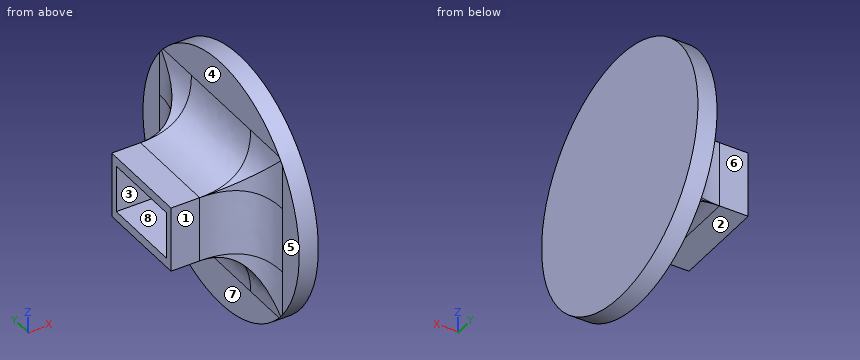
from build123d import *

# Parameters (mm, degrees)
SKETCH2_R           = 19.65
BOSS_EXTRUDE1_DEPTH = 3
SKETCH3_W           = 12.5
SKETCH3_H           = 14.9
BOSS_EXTRUDE2_DEPTH = 5.15
SKETCH4_W           = 7.4
SKETCH4_H           = 12.6
CUT_EXTRUDE1_DEPTH  = 12.5
FILLET1_SIZE        = 8


with BuildPart() as part:
    # Sketch2 → Boss-Extrude1 (new body)
    with BuildSketch(Plane(origin=(0, 0, 0), x_dir=(0, 0, -1), z_dir=(1, 0, 0))):
        Circle(SKETCH2_R)
    extrude(amount=BOSS_EXTRUDE1_DEPTH)

    # Sketch3 → Boss-Extrude2 (add, symmetric)
    with BuildSketch(Plane.XY):
        with Locations((-6.25, 0)):
            Rectangle(SKETCH3_W, SKETCH3_H)
    extrude(amount=BOSS_EXTRUDE2_DEPTH, both=True)

    # Sketch4 → Cut-Extrude1 (cut)
    with BuildSketch(Plane.ZY.offset(12.5)):
        Rectangle(SKETCH4_W, SKETCH4_H)
    extrude(amount=-CUT_EXTRUDE1_DEPTH, mode=Mode.SUBTRACT)

    # Fillet1
    # a fillet whose section is not a circle: 8 mm, written as the material it adds along each edge
    with BuildSketch(Plane(origin=(0, 7.45, 5.15), x_dir=(0, 1, 0), z_dir=(0, 0, -1))) as fillet1_piece_1:
        with BuildLine():
            Bezier((FILLET1_SIZE, 0), (0, 0), (0, -FILLET1_SIZE), weights=[1, 1, 1])
            Line((0, -FILLET1_SIZE), (0, 0))
            Line((0, 0), (FILLET1_SIZE, 0))
        make_face()
    extrude(amount=10.3)
    with BuildSketch(Plane(origin=(0, -7.45, 5.15), x_dir=(0, 0, 1), z_dir=(0, 1, 0))) as fillet1_piece_2:
        with BuildLine():
            Bezier((FILLET1_SIZE, 0), (0, 0), (0, -FILLET1_SIZE), weights=[1, 1, 1])
            Line((0, -FILLET1_SIZE), (0, 0))
            Line((0, 0), (FILLET1_SIZE, 0))
        make_face()
    extrude(amount=14.9)
    with BuildSketch(Plane(origin=(0, -7.45, 5.15), x_dir=(0, -1, 0), z_dir=(0, 0, -1))) as fillet1_piece_3:
        with BuildLine():
            Bezier((FILLET1_SIZE, 0), (0, 0), (0, FILLET1_SIZE), weights=[1, 1, 1])
            Line((0, FILLET1_SIZE), (0, 0))
            Line((0, 0), (FILLET1_SIZE, 0))
        make_face()
    extrude(amount=10.3)
    with BuildSketch(Plane(origin=(0, -7.45, -5.15), x_dir=(0, 0, -1), z_dir=(0, 1, 0))) as fillet1_piece_4:
        with BuildLine():
            Bezier((FILLET1_SIZE, 0), (0, 0), (0, FILLET1_SIZE), weights=[1, 1, 1])
            Line((0, FILLET1_SIZE), (0, 0))
            Line((0, 0), (FILLET1_SIZE, 0))
        make_face()
    extrude(amount=14.9)
    with BuildSketch(Plane(origin=(0, -7.45, 5.15), x_dir=(0, 0, 1), z_dir=(0, 1, 0))) as fillet1_piece_5a_section:
        with BuildLine():
            Bezier((FILLET1_SIZE, 0), (0, 0), (0, -FILLET1_SIZE), weights=[1, 1, 1])
            Line((0, -FILLET1_SIZE), (0, 0))
            Line((0, 0), (FILLET1_SIZE, 0))
        make_face()
    fillet1_piece_5a = extrude(amount=34.9, mode=Mode.PRIVATE)
    fillet1_piece_5a = fillet1_piece_5a & Plane(origin=(0, 0, 0), x_dir=(0, 0, -1), z_dir=(-1, 0, 0)) * Cylinder(19.65, 102, mode=Mode.PRIVATE)
    fillet1_piece_5a = split(fillet1_piece_5a, bisect_by=Plane(origin=(0, 7.45, 5.15), z_dir=(0, 1, 0)), keep=Keep.TOP, mode=Mode.PRIVATE)
    with BuildSketch(Plane(origin=(0, 7.45, 25.15), x_dir=(0, 1, 0), z_dir=(0, 0, -1))) as fillet1_piece_5b_section:
        with BuildLine():
            Bezier((FILLET1_SIZE, 0), (0, 0), (0, -FILLET1_SIZE), weights=[1, 1, 1])
            Line((0, -FILLET1_SIZE), (0, 0))
            Line((0, 0), (FILLET1_SIZE, 0))
        make_face()
    fillet1_piece_5b = extrude(amount=30.3, mode=Mode.PRIVATE)
    fillet1_piece_5b = fillet1_piece_5b & Plane(origin=(0, 0, 0), x_dir=(0, 0, -1), z_dir=(-1, 0, 0)) * Cylinder(19.65, 93, mode=Mode.PRIVATE)
    fillet1_piece_5b = split(fillet1_piece_5b, bisect_by=Plane(origin=(0, 7.45, 5.15), z_dir=(0, 0, 1)), keep=Keep.TOP, mode=Mode.PRIVATE)
    fillet1_piece_5 = fillet1_piece_5a & fillet1_piece_5b
    add(fillet1_piece_5)
    with BuildSketch(Plane(origin=(0, -7.45, -5.15), x_dir=(0, 0, -1), z_dir=(0, 1, 0))) as fillet1_piece_6a_section:
        with BuildLine():
            Bezier((FILLET1_SIZE, 0), (0, 0), (0, FILLET1_SIZE), weights=[1, 1, 1])
            Line((0, FILLET1_SIZE), (0, 0))
            Line((0, 0), (FILLET1_SIZE, 0))
        make_face()
    fillet1_piece_6a = extrude(amount=34.9, mode=Mode.PRIVATE)
    fillet1_piece_6a = fillet1_piece_6a & Plane(origin=(0, 0, 0), x_dir=(0, 0, -1), z_dir=(-1, 0, 0)) * Cylinder(19.65, 102, mode=Mode.PRIVATE)
    fillet1_piece_6a = split(fillet1_piece_6a, bisect_by=Plane(origin=(0, 7.45, -5.15), z_dir=(0, 1, 0)), keep=Keep.TOP, mode=Mode.PRIVATE)
    with BuildSketch(Plane(origin=(0, 7.45, 5.15), x_dir=(0, 1, 0), z_dir=(0, 0, -1))) as fillet1_piece_6b_section:
        with BuildLine():
            Bezier((FILLET1_SIZE, 0), (0, 0), (0, -FILLET1_SIZE), weights=[1, 1, 1])
            Line((0, -FILLET1_SIZE), (0, 0))
            Line((0, 0), (FILLET1_SIZE, 0))
        make_face()
    fillet1_piece_6b = extrude(amount=30.3, mode=Mode.PRIVATE)
    fillet1_piece_6b = fillet1_piece_6b & Plane(origin=(0, 0, 0), x_dir=(0, 0, -1), z_dir=(-1, 0, 0)) * Cylinder(19.65, 93, mode=Mode.PRIVATE)
    fillet1_piece_6b = split(fillet1_piece_6b, bisect_by=Plane(origin=(0, 7.45, -5.15), z_dir=(0, 0, -1)), keep=Keep.TOP, mode=Mode.PRIVATE)
    fillet1_piece_6 = fillet1_piece_6a & fillet1_piece_6b
    add(fillet1_piece_6)
    with BuildSketch(Plane(origin=(0, -27.45, 5.15), x_dir=(0, 0, 1), z_dir=(0, 1, 0))) as fillet1_piece_7a_section:
        with BuildLine():
            Bezier((FILLET1_SIZE, 0), (0, 0), (0, -FILLET1_SIZE), weights=[1, 1, 1])
            Line((0, -FILLET1_SIZE), (0, 0))
            Line((0, 0), (FILLET1_SIZE, 0))
        make_face()
    fillet1_piece_7a = extrude(amount=34.9, mode=Mode.PRIVATE)
    fillet1_piece_7a = fillet1_piece_7a & Plane(origin=(0, 0, 0), x_dir=(0, 0, -1), z_dir=(-1, 0, 0)) * Cylinder(19.65, 102, mode=Mode.PRIVATE)
    fillet1_piece_7a = split(fillet1_piece_7a, bisect_by=Plane(origin=(0, -7.45, 5.15), z_dir=(0, -1, 0)), keep=Keep.TOP, mode=Mode.PRIVATE)
    with BuildSketch(Plane(origin=(0, -7.45, 25.15), x_dir=(0, -1, 0), z_dir=(0, 0, -1))) as fillet1_piece_7b_section:
        with BuildLine():
            Bezier((FILLET1_SIZE, 0), (0, 0), (0, FILLET1_SIZE), weights=[1, 1, 1])
            Line((0, FILLET1_SIZE), (0, 0))
            Line((0, 0), (FILLET1_SIZE, 0))
        make_face()
    fillet1_piece_7b = extrude(amount=30.3, mode=Mode.PRIVATE)
    fillet1_piece_7b = fillet1_piece_7b & Plane(origin=(0, 0, 0), x_dir=(0, 0, -1), z_dir=(-1, 0, 0)) * Cylinder(19.65, 93, mode=Mode.PRIVATE)
    fillet1_piece_7b = split(fillet1_piece_7b, bisect_by=Plane(origin=(0, -7.45, 5.15), z_dir=(0, 0, 1)), keep=Keep.TOP, mode=Mode.PRIVATE)
    fillet1_piece_7 = fillet1_piece_7a & fillet1_piece_7b
    add(fillet1_piece_7)
    with BuildSketch(Plane(origin=(0, -7.45, 5.15), x_dir=(0, -1, 0), z_dir=(0, 0, -1))) as fillet1_piece_8a_section:
        with BuildLine():
            Bezier((FILLET1_SIZE, 0), (0, 0), (0, FILLET1_SIZE), weights=[1, 1, 1])
            Line((0, FILLET1_SIZE), (0, 0))
            Line((0, 0), (FILLET1_SIZE, 0))
        make_face()
    fillet1_piece_8a = extrude(amount=30.3, mode=Mode.PRIVATE)
    fillet1_piece_8a = fillet1_piece_8a & Plane(origin=(0, 0, 0), x_dir=(0, 0, -1), z_dir=(-1, 0, 0)) * Cylinder(19.65, 93, mode=Mode.PRIVATE)
    fillet1_piece_8a = split(fillet1_piece_8a, bisect_by=Plane(origin=(0, -7.45, -5.15), z_dir=(0, 0, -1)), keep=Keep.TOP, mode=Mode.PRIVATE)
    with BuildSketch(Plane(origin=(0, -27.45, -5.15), x_dir=(0, 0, -1), z_dir=(0, 1, 0))) as fillet1_piece_8b_section:
        with BuildLine():
            Bezier((FILLET1_SIZE, 0), (0, 0), (0, FILLET1_SIZE), weights=[1, 1, 1])
            Line((0, FILLET1_SIZE), (0, 0))
            Line((0, 0), (FILLET1_SIZE, 0))
        make_face()
    fillet1_piece_8b = extrude(amount=34.9, mode=Mode.PRIVATE)
    fillet1_piece_8b = fillet1_piece_8b & Plane(origin=(0, 0, 0), x_dir=(0, 0, -1), z_dir=(-1, 0, 0)) * Cylinder(19.65, 102, mode=Mode.PRIVATE)
    fillet1_piece_8b = split(fillet1_piece_8b, bisect_by=Plane(origin=(0, -7.45, -5.15), z_dir=(0, -1, 0)), keep=Keep.TOP, mode=Mode.PRIVATE)
    fillet1_piece_8 = fillet1_piece_8a & fillet1_piece_8b
    add(fillet1_piece_8)


solid = part.part
Model file for the job. Use its own axes, mm. Face numbers are marked on the shaded views. A direction names the side the tool comes from. Coordinates: 2 decimals unless noted, no trailing zeros. Write each loop counter-clockwise with the first axis right and the second up, starting at its lowest first coordinate (ties: lowest second). Pieces come first, ordered by that corner, then holes. Notation, with made-up numbers: (34.5, 78.5) -> (75.5, 78.5) arc R21 cw to (75.5, 111.5) -> close; hole circle Ø8 at (86, 13). An arc over 180 degrees is marked (long way). One line per item, written item: value. Start each with the question number.
1) Slice it at A-A on x = -10.5. Write the cut outline in (y, z).
2) Which spindle directions (+Z, -Z, +X, -X, +Y, -Y) get a long thin tool onto all of the face, cutting with end or side? Do the marked faces 4, 5, 6, 7 and 8. Say none if no direction does.
3) Flat gauge pins, fed straight in: pin 1 Ø5 at (x, z) = (-10.5, 1) entering from -Y; pin 2 Ø6 at (y, z) = (10.5, -14) entering from -X; pin 3 Ø5 at (x, y) = (-9.5, -3) entering from +Z. Where does each tip first touch, or does it go through?
4) Pull direction Y, two halves, no side cores. Call the marked faces 1, 2 and 3: +Y half, -Y half, draft (parallel to the pull), parting line (faces both ways), or undercut.
5) Probe probe 1 along Y at (x, z) = (-7.5, 0.5); probe 2 along Z at (x, y) = (-9, 6); probe 3 along X at (y, z) = (-3, -16.5). List the from-to ranges inside material, lowest first.
6) Slice it at B-B on z = -16. Write the cut outline in (x, y).
Answers follow:
1. outline: (-7.45, -5.15) -> (7.45, -5.15) -> (7.45, 5.15) -> (-7.45, 5.15) -> close; hole (-6.3, -3.7) -> (6.3, -3.7) -> (6.3, 3.7) -> (-6.3, 3.7) -> close
2. face 4: +Z, -X, +Y, -Y
2. face 5: +Z, -Z, -X, -Y
2. face 6: +Z, -Z, -X, +Y
2. face 7: -Z, -X, +Y, -Y
2. face 8: -X
3. pin 1: y = -7.45
3. pin 2: x = -0.17
3. pin 3: z = 5.18
4. face 1: -Y half
4. face 2: draft
4. face 3: undercut
5. probe 1: -7.46 to -6.3, 6.3 to 7.46
5. probe 2: -5.15 to -3.7, 3.7 to 5.15
5. probe 3: 0 to 3
6. outline: (0, -11.41) -> (3, -11.41) -> (3, 11.41) -> (0, 11.41) -> close
